The drawing under review shows one solid part. Ordinate dimensions are in mm from its lowest x, y, z. Coordinates: 2 decimals unless noted, no trailing zeros. Order: outer loops, then holes, each group sorted by start corner. A loop starts at its lowest first (then second) coordinate and runs counter-clockwise, first axis right, second up. Notation, with made-up numbers: (69.25, 34) -> (122.25, 34) arc R27 cw to (122.25, 63) -> close; hole circle Ø8 at (13.5, 59). An arc over 180 degrees is marked (long way). Write item = value, one per line.
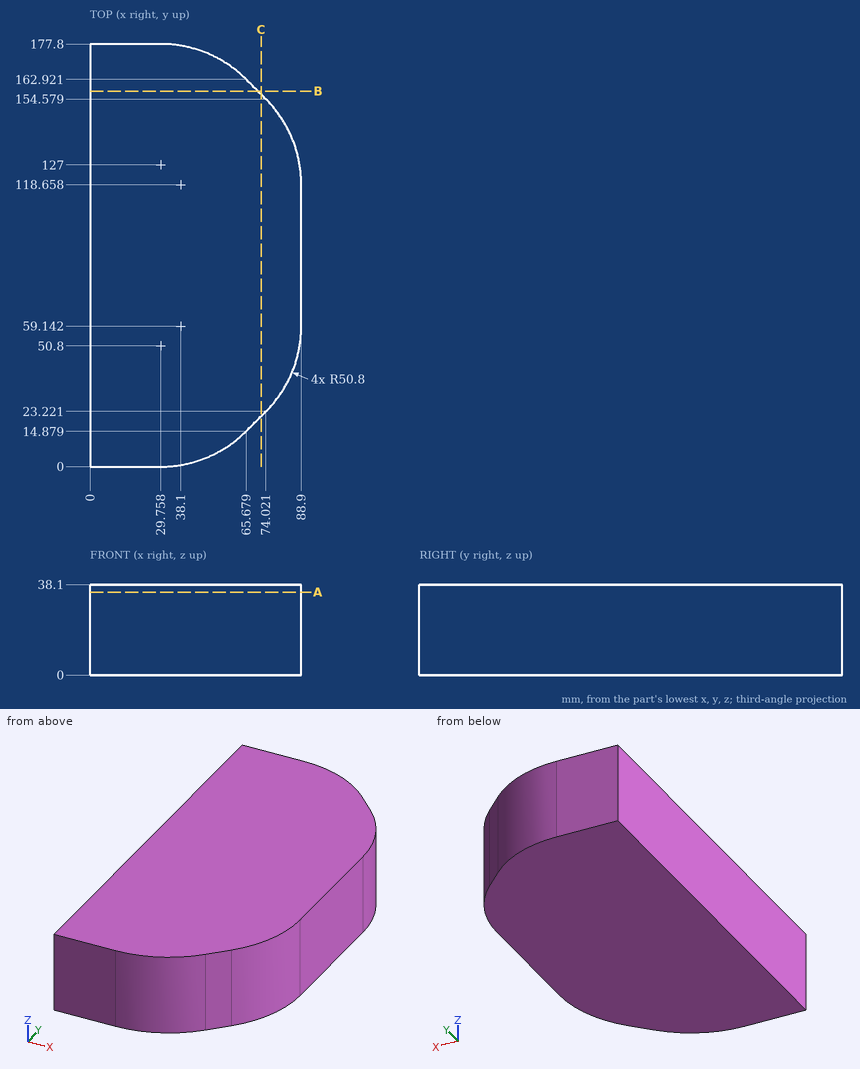
(1) For L1, parallel to Y at x = 46, z = 2.5; L2, parallel to Y at x = 59, z = 15; L3, parallel to X at y = 134, z = 30, list the stretches that pass through material, from the lowest coordinate up.
Report:
L1 = 2.67 to 175.13
L2 = 9.26 to 168.54
L3 = 0 to 86.53
(2) Insertion check: pin 1 (5 mm diameter, centred on y = 151.5, z = 29.5, fed in from +X); pin 2 (5 mm diameter, centred on x = 69, z = 30.5, fed in from -Y); pin 3 (4 mm diameter, centred on x = 59, z = 7, fed in from +Y); pin 4 (12 mm diameter, centred on x = 47.5, y = 65.5, fed in from -Z). Each pin has a flat end and moves straight along its axis. Give the tip position at first contact, or say it passes through.
Report:
pin_1 = 78.84
pin_2 = 15.7
pin_3 = 169.88
pin_4 = 0
(3) We need section A-A (z = 35). Write out the cut boundary in (x, y), and give its area (3 significant figures).
Report:
outline = (0, 0) -> (29.76, 0) arc R50.8 ccw to (65.68, 14.88) -> (74.02, 23.22) arc R50.8 ccw to (88.9, 59.14) -> (88.9, 118.66) arc R50.8 ccw to (74.02, 154.58) -> (65.68, 162.92) arc R50.8 ccw to (29.76, 177.8) -> (0, 177.8) -> close
area = 14,100 mm²
(4) We need section C-C (x = 72). Write out the cut boundary in (y, z).
Report:
outline = (21.2, 0) -> (156.6, 0) -> (156.6, 38.1) -> (21.2, 38.1) -> close
(5) We need section B-B (y = 158). Write out the cut boundary in (x, z).
Report:
outline = (0, 0) -> (70.6, 0) -> (70.6, 38.1) -> (0, 38.1) -> close
